Build history of the part. All positions in model axes, mm. A direction names the side the tool comes from. Coordinates: 2 decimals unless noted, no trailing zeros. Loops run counter-clockwise (first coordinate to the right, second up) from the corner with the lowest first, then second, coordinate; pieces in that order, holes last. Notation, with made-up numbers: (83.25, 64.5) -> (108.25, 64.5) arc R13 ccw to (108.25, 81.5) -> close; hole circle Ø9 at (32, 24). An arc over 180 degrees is marked (long way). One line per item, written item: value. Start each with the question number.
```python
from build123d import *

# Parameters (mm, degrees)
BOSS_EXTRUDE1_DEPTH   = 6.35
M4X0_7_TAPPED_HOLE1_D = 3.3
MOVE_START            = -1.5452
MOVE_FACE1_DEPTH      = 6.35
FILLET1_R             = 0.762
CHAMFER1_SIZE         = 0.254


# Read off the part's stored shape, not the designer's step: Move Face1
with BuildPart() as part:
    # Sketch1 → Boss-Extrude1 (new body)
    with BuildSketch(Plane(origin=(0, -1.5452, 0), x_dir=(1, 0, 0), z_dir=(0, 1, 0))):
        with BuildLine():
            Line((-38.502216327, 6.405933187), (-37.466084693, -13.910736196))
            ThreePointArc((-37.466084693, -13.910736196), (0, -49.514775956), (37.466084693, -13.910736196))
            Line((37.466084693, -13.910736196), (38.502216327, 6.405933187))
            ThreePointArc((38.502216327, 6.405933187), (37.384487444, 9.425866669), (34.42540277, 10.695958786))
            Line((34.42540277, 10.695958786), (32.657493289, 10.695958786))
            ThreePointArc((32.657493289, 10.695958786), (32.454748459, 10.594968738), (32.41333978, 10.372281116))
            Line((32.41333978, 10.372281116), (36.356433895, -3.429162442))
            ThreePointArc((36.356433895, -3.429162442), (36.223319367, -4.587824739), (35.309857101, -5.312948512))
            Line((35.309857101, -5.312948512), (30.453700202, -6.70036017))
            Line((30.453700202, -6.70036017), (30.10512277, -13.535333842))
            ThreePointArc((30.10512277, -13.535333842), (0, -42.14424766), (-30.10512277, -13.535333842))
            Line((-30.10512277, -13.535333842), (-30.453700202, -6.70036017))
            Line((-30.453700202, -6.70036017), (-35.309857101, -5.312948512))
            ThreePointArc((-35.309857101, -5.312948512), (-36.223319367, -4.587824739), (-36.356433895, -3.429162442))
            Line((-36.356433895, -3.429162442), (-32.41333978, 10.372281116))
            ThreePointArc((-32.41333978, 10.372281116), (-32.454748459, 10.594968738), (-32.657493289, 10.695958786))
            Line((-32.657493289, 10.695958786), (-34.42540277, 10.695958786))
            ThreePointArc((-34.42540277, 10.695958786), (-37.384487444, 9.425866669), (-38.502216327, 6.405933187))
        make_face()
    extrude(amount=BOSS_EXTRUDE1_DEPTH)

    # M4x0.7 Tapped Hole1 (through all)
    with Locations(Plane(origin=(0, -1.5452, 0), x_dir=(-1, 0, 0), z_dir=(0, -1, 0))):
        with Locations((31.804908667, -22.86), (35.794080898, 7.112), (0, -45.607912987), (-31.804908667, -22.86), (-35.794080898, 7.112)):
            Hole(M4X0_7_TAPPED_HOLE1_D / 2)

    # Move Face1 outline → Move Face1 (add)
    with BuildSketch(Plane(origin=(0, 0, 0), x_dir=(1, 0, 0), z_dir=(0, 1, 0)).offset(MOVE_START)):
        with BuildLine():
            ThreePointArc((-34.42540277, 11.330958786), (-37.844793004, 9.863295282), (-39.136392147, 6.373590798))
            Line((-39.136392147, 6.373590798), (-38.100260512, -13.943078585))
            ThreePointArc((-38.100260512, -13.943078585), (0, -50.149775956), (38.100260512, -13.943078585))
            Line((38.100260512, -13.943078585), (39.136392147, 6.373590798))
            ThreePointArc((39.136392147, 6.373590798), (37.844793004, 9.863295282), (34.42540277, 11.330958786))
            Line((34.42540277, 11.330958786), (32.657662642, 11.330958764))
            ThreePointArc((32.657662642, 11.330958764), (31.94785031, 10.977433467), (31.802770017, 10.197840375))
            Line((31.802770017, 10.197840375), (35.745873307, -3.603635272))
            ThreePointArc((35.745873307, -3.603635272), (35.668225017, -4.27944954), (35.135416361, -4.702378753))
            Line((35.135416361, -4.702378753), (29.842651852, -6.214529893))
            Line((29.842651852, -6.214529893), (29.47094695, -13.502991453))
            ThreePointArc((29.47094695, -13.502991453), (0, -41.50924766), (-29.47094695, -13.502991453))
            Line((-29.47094695, -13.502991453), (-29.842651852, -6.214529893))
            Line((-29.842651852, -6.214529893), (-35.135448453, -4.702369587))
            ThreePointArc((-35.135448453, -4.702369587), (-35.668241226, -4.279420366), (-35.745864137, -3.603603182))
            Line((-35.745864137, -3.603603182), (-31.802816567, 10.197677545))
            ThreePointArc((-31.802816567, 10.197677545), (-31.947748326, 10.977298265), (-32.657493289, 11.330958793))
            Line((-32.657493289, 11.330958793), (-34.42540277, 11.330958786))
        make_face()
        with BuildLine():
            Line((-37.466084693, -13.910736196), (-38.502216327, 6.405933187))
            ThreePointArc((-38.502216327, 6.405933187), (-37.384487444, 9.425866669), (-34.42540277, 10.695958786))
            Line((-34.42540277, 10.695958786), (-32.657493289, 10.695958786))
            ThreePointArc((-32.657493289, 10.695958786), (-32.454748459, 10.594968738), (-32.41333978, 10.372281116))
            Line((-32.41333978, 10.372281116), (-36.356433895, -3.429162442))
            ThreePointArc((-36.356433895, -3.429162442), (-36.223319367, -4.587824739), (-35.309857101, -5.312948512))
            Line((-35.309857101, -5.312948512), (-30.453700202, -6.70036017))
            Line((-30.453700202, -6.70036017), (-30.10512277, -13.535333842))
            ThreePointArc((-30.10512277, -13.535333842), (0, -42.14424766), (30.10512277, -13.535333842))
            Line((30.10512277, -13.535333842), (30.453700202, -6.70036017))
            Line((30.453700202, -6.70036017), (35.309857101, -5.312948512))
            ThreePointArc((35.309857101, -5.312948512), (36.223319367, -4.587824739), (36.356433895, -3.429162442))
            Line((36.356433895, -3.429162442), (32.41333978, 10.372281116))
            ThreePointArc((32.41333978, 10.372281116), (32.454748459, 10.594968738), (32.657493289, 10.695958786))
            Line((32.657493289, 10.695958786), (34.42540277, 10.695958786))
            ThreePointArc((34.42540277, 10.695958786), (37.384487444, 9.425866669), (38.502216327, 6.405933187))
            Line((38.502216327, 6.405933187), (37.466084693, -13.910736196))
            ThreePointArc((37.466084693, -13.910736196), (0, -49.514775956), (-37.466084693, -13.910736196))
        make_face(mode=Mode.SUBTRACT)
    extrude(amount=MOVE_FACE1_DEPTH)

    # Fillet1
    fillet1_edges = [part.edges().sort_by_distance(p)[0] for p in [
        (-29.842651852, 1.6298, 6.214529893),
        (29.842651852, 1.6298, 6.214529893),
    ]]
    fillet(fillet1_edges, radius=FILLET1_R)

    # Chamfer1
    chamfer1_edges = [part.edges().sort_by_distance(p)[0] for p in [
        (0, 4.8048, 50.149775956),
        (38.61832633, 4.8048, 3.784743893),
        (-33.54144803, -1.5452, -11.33095879),
        (37.844793004, 4.8048, -9.863295282),
        (-31.947748326, -1.5452, -10.977298265),
        (-33.774340352, -1.5452, -3.297037181),
        (-35.668241226, -1.5452, 4.279420366),
        (-29.642922919, -1.5452, 10.130853406),
        (0, -1.5452, 41.50924766),
        (32.750998673, -1.5452, 5.383610635),
        (33.541532706, 4.8048, -11.330958775),
        (35.668225017, -1.5452, 4.27944954),
        (33.774321662, -1.5452, -3.297102552),
        (31.94785031, -1.5452, -10.977433467),
        (33.541532706, -1.5452, -11.330958775),
        (37.844793004, -1.5452, -9.863295282),
        (38.61832633, -1.5452, 3.784743893),
        (0, -1.5452, 50.149775956),
        (31.94785031, 4.8048, -10.977433467),
        (-38.61832633, -1.5452, 3.784743893),
        (-37.844793004, -1.5452, -9.863295282),
        (33.774321662, 4.8048, -3.297102552),
        (35.668225017, 4.8048, 4.27944954),
        (32.750998673, 4.8048, 5.383610635),
        (0, 4.8048, 41.50924766),
        (-37.844793004, 4.8048, -9.863295282),
        (-29.642922919, 4.8048, 10.130853406),
        (-35.668241226, 4.8048, 4.279420366),
        (-33.774340352, 4.8048, -3.297037181),
        (-31.947748326, 4.8048, -10.977298265),
        (34.144080898, -1.5452, -7.112),
        (34.144080898, 4.8048, -7.112),
        (-33.54144803, 4.8048, -11.33095879),
        (30.154908667, -1.5452, 22.86),
        (30.154908667, 4.8048, 22.86),
        (-1.65, -1.5452, 45.607912987),
        (-1.65, 4.8048, 45.607912987),
        (-37.444080898, -1.5452, -7.112),
        (-37.444080898, 4.8048, -7.112),
        (-38.61832633, 4.8048, 3.784743893),
        (-33.454908667, -1.5452, 22.86),
        (-33.454908667, 4.8048, 22.86),
        (-32.751014719, -1.5452, 5.383606052),
        (-32.751014719, 4.8048, 5.383606052),
        (29.642922919, -1.5452, 10.130853405),
        (29.979458075, -1.5452, 6.323301327),
        (-29.979458075, -1.5452, 6.323301327),
        (29.642922919, 4.8048, 10.130853405),
        (29.979458075, 4.8048, 6.323301327),
        (-29.979458075, 4.8048, 6.323301327),
    ]]
    chamfer(chamfer1_edges, length=CHAMFER1_SIZE)


solid = part.part
```
Item 1: Band-saw the part on C-C, the plane y = 2.75. List the corners of the cut face in (x, z).
Item 2: Band-saw the part on A-A, the plane x = 0. List the corners of the cut face in (y, z), and give its area (3 significant figures).
Item 3: Probe probe 1 along Z at (x, y) = (0, 1.9); probe 2 along X at (y, z) = (-1, -7); probe 3 along X at (y, z) = (-1.25, 23). List the from-to ranges inside material, lowest first.
Item 4: Tool access for faces 1 (the face through (-38.626, 1.589, 3.643)), 2 (the face through (-33.922, -1.416, -3.235)), 3 (the face through (-32.75, 4.68, 5.52)): list every direction of +Z, -Z, +X, -X, +Y, -Y with a clear straight run to the whole face (end or side of a thin tool).
Item 5: Drop flat-ended pins along their axis: pin 1 Ø2 at (x, z) = (31.8, 22.86) entering from -Y; pin 2 Ø1.5 at (x, y) = (30, 0) entering from +Z; pin 3 Ø2 at (y, z) = (3, 24.5) entering from +X. Give the stop position or say it passes through.
Item 6: Two-plate mould, pull along X, no slides. Class faces 4 (the face through (38.61, 1.59, 3.93)), 5 (the face through (-32.7, 1.6, 5.4)), 6 (the face through (-37.72, 4.68, -9.81)): +X half, -X half, draft (parallel to the pull), parting line (faces both ways), or undercut.
Item 7: Band-saw the part on D-D, the plane z = 22.86. Count the separate pieces of the cut face and the enclosed holes in it, and give its area (3 significant figures).
Item 8: Band-saw the part on B-B, the plane z = 12. List the corners of the cut face in (x, y), and give its area (3 significant figures).
Worked out:
1. outline: (-39.14, -6.37) arc R4.72 ccw to (-34.43, -11.33) -> (-32.66, -11.33) arc R0.89 ccw to (-31.8, -10.2) -> (-35.75, 3.6) arc R0.89 cw to (-35.14, 4.7) -> (-30.37, 6.06) arc R0.76 ccw to (-29.81, 6.76) -> (-29.47, 13.5) arc R29.51 cw to (29.47, 13.5) -> (29.81, 6.76) arc R0.76 ccw to (30.37, 6.06) -> (35.14, 4.7) arc R0.89 cw to (35.75, 3.6) -> (31.8, -10.2) arc R0.89 ccw to (32.66, -11.33) -> (34.43, -11.33) arc R4.72 ccw to (39.14, -6.37) -> (38.1, 13.94) arc R38.15 ccw to (-38.1, 13.94) -> close; hole circle Ø3.3 at (-35.79, -7.11); hole circle Ø3.3 at (-31.8, 22.86); hole circle Ø3.3 at (0, 45.61); hole circle Ø3.3 at (31.8, 22.86); hole circle Ø3.3 at (35.79, -7.11)
2. outline: (-1.55, 41.76) -> (-1.29, 41.51) -> (4.55, 41.51) -> (4.8, 41.76) -> (4.8, 43.7) -> (4.55, 43.96) -> (-1.29, 43.96) -> (-1.55, 43.7) -> close; (-1.55, 47.51) -> (-1.29, 47.26) -> (4.55, 47.26) -> (4.8, 47.51) -> (4.8, 49.9) -> (4.55, 50.15) -> (-1.29, 50.15) -> (-1.55, 49.9) -> close
2. area: 33.7 mm²
3. probe 1: z = 41.51 to 43.96, 47.26 to 50.15
3. probe 2: x = -39.13 to -37.44, -34.15 to -32.72, 32.72 to 34.15, 37.44 to 39.13
3. probe 3: x = -36.53 to -33.45, -30.16 to -27.38, 27.38 to 30.16, 33.45 to 36.53
4. face 1: +Z, -X, +Y, -Y
4. face 2: -Y
4. face 3: +Y
5. pin 1: passes through
5. pin 2: stops at z = 36.49
5. pin 3: stops at x = 36.38
6. face 4: +X half
6. face 5: undercut
6. face 6: -X half
7. separate pieces: 4
7. enclosed holes: 0
7. area: 73.5 mm²
8. outline: (-38.2, -1.29) -> (-37.95, -1.55) -> (-29.8, -1.55) -> (-29.55, -1.29) -> (-29.55, 4.55) -> (-29.8, 4.8) -> (-37.95, 4.8) -> (-38.2, 4.55) -> close; (29.55, -1.29) -> (29.8, -1.55) -> (37.95, -1.55) -> (38.2, -1.29) -> (38.2, 4.55) -> (37.95, 4.8) -> (29.8, 4.8) -> (29.55, 4.55) -> close
8. area: 110 mm²
